```python
from build123d import *

# Parameters (mm, degrees)
SKIZZE3_W                       = 1.5
SKIZZE3_H                       = 14
SCHNITT_LINEAR_AUSTRAGEN2_DEPTH = 3
VERRUNDUNG1_R                   = 0.6
VERRUNDUNG3_R                   = 0.6


with BuildPart() as part:
    # Skizze1 → Rotation1 (revolve)
    with BuildSketch(Plane.XY):
        Polygon((-3, 0), (-3, 6), (-2, 7), (0, 7), (0, 4), (30, 4), (30, 2.2), (32.114359354, 2.2), (33.5, 3), (40.5, 3), (41, 2.711324865), (41, 0), align=None)
    revolve(axis=Axis((41, 0, 0), (-1, 0, 0)))

    # Skizze3 → Schnitt-Linear austragen2 (cut)
    with BuildSketch(Plane(origin=(0, 0, 0), x_dir=(0, 0, -1), z_dir=(1, 0, 0))):
        with Locations((-6.25, 0)):
            Rectangle(SKIZZE3_W, SKIZZE3_H)
        with Locations((6.25, 0)):
            Rectangle(SKIZZE3_W, SKIZZE3_H)
    extrude(amount=-SCHNITT_LINEAR_AUSTRAGEN2_DEPTH, mode=Mode.SUBTRACT)

    # Verrundung1
    verrundung1_edges = [part.edges().sort_by_distance(p)[0] for p in [
        (0, -4, 0),
    ]]
    fillet(verrundung1_edges, radius=VERRUNDUNG1_R)

    # Verrundung3
    verrundung3_edges = [part.edges().sort_by_distance(p)[0] for p in [
        (32.114359354, -2.2, 0),
        (30, -2.2, 0),
    ]]
    fillet(verrundung3_edges, radius=VERRUNDUNG3_R)


solid = part.part
```
Part model, mm, in its own coordinate system. A direction names the side the tool comes from. Round coordinates to 2 decimals unless told otherwise and drop trailing zeros. Loops run counter-clockwise (first coordinate to the right, second up) from the corner with the lowest first, then second, coordinate; pieces in that order, holes last. Notation, with made-up numbers: (89, -28.75) -> (145, -28.75) arc R10 cw to (145, -22.75) -> close; hole circle Ø5 at (1.5, -5). An arc over 180 degrees is marked (long way). Use a Markdown table: item, result.
1) Drop flat-ended pins along their axis: pin 1 Ø1.5 at (x, y) = (10, -1.5) entering from +Z; pin 2 Ø1.5 at (x, z) = (23, -0.5) entering from -Y; pin 3 Ø2 at (x, y) = (9, -4.5) entering from -Z. Give the stop position or say it passes through.
The answers:
| item | result |
|---|---|
| pin 1 | stops at z = 3.93 |
| pin 2 | stops at y = -4 |
| pin 3 | stops at z = -1.94 |
2) Tool access for faces 4 (the flat face through (30, 1, -3)), 5 (the cylindrical face through (15.506, -0.867, 3.905)), 6 (the flat face through (-1, 0, -5.5)): list every direction of +Z, -Z, +X, -X, +Y, -Y with a clear straight run to the whole face (end or side of a thin tool).
The answers:
| item | result |
|---|---|
| face 4 | none |
| face 5 | +X |
| face 6 | -Z, +X, -X, +Y, -Y |
3) Cut at A-A, the plane x = 36. List the corners of the cut face in (y, z), and give its area (3 significant figures).
The answers:
| item | result |
|---|---|
| outline | circle Ø6 at (0, 0) |
| area | 28.3 mm2 |
4) Probe line 1 (X direction, y = 3.5, z = -1.5); line 2 (X direction, y = -3.5, z = 4.5); line 3 (Y direction, x = 25, z = -1). List the from-to ranges inside material, lowest first. Write a range as [from, to].
The answers:
| item | result |
|---|---|
| line 1 | x = [-3, 30] |
| line 2 | x = [-3, 0] |
| line 3 | y = [-3.87, 3.87] |
5) Cut at B-B, the plane x = 21.5. List the corners of the cut face in (y, z), and give its area (3 significant figures).
The answers:
| item | result |
|---|---|
| outline | circle Ø8 at (0, 0) |
| area | 50.3 mm2 |
6) Pull direction X, two halves, no side cores. Call faces 1 (the conical face through (-2.8, 6.2, 0.1)), 2 (the cylindrical face through (-1, 7, 0)), 3 (the cylindrical face through (31.29, 2.1, -0.66)): pulls with the +X half, pulls with the -X half, needs draft (parallel to the pull), parting line crosses it, or undercut.
The answers:
| item | result |
|---|---|
| face 1 | pulls with the -X half |
| face 2 | needs draft |
| face 3 | undercut |
